Input: part model. Units: mm. Frame: model coordinates. A direction names the side the tool comes from. Coordinates: 2 decimals unless noted, no trailing zeros. Write each loop counter-clockwise with the first axis right and the second up, starting at its lowest first coordinate (ties: lowest second). Pieces come first, ordered by that corner, then holes.
1) Draft query along Y for faces 1 (the flat face through (21, 0, 21)), 2 (the cylindrical face through (16.16, -14.47, 37.88)), 3 (the cylindrical face through (-2.38, -10.74, 41.09)). Return one class per face: pulls with the +Y half, pulls with the -Y half, needs draft (parallel to the pull), parting line crosses it, or undercut.
2) Set-up query: faces 4 (the flat face through (15, -16, 3)), 5 (the flat face through (23, -8.2, 41)), 6 (the cylindrical face through (16.16, 16.53, 37.88)). Return all of +Z, -Z, +X, -X, +Y, -Y with unobstructed straight access to the full face (end or side cutting, diameter ignored); none if empty.
3) Pin query (flat end, axial travel): pin 1 Ø4.5 at (x, y) = (23.5, 3) entering from -Z; pin 2 Ø3 at (x, z) = (22.5, 42) entering from -Y; pin 3 Ø5 at (x, z) = (17, 39.5) entering from +Y; pin 4 Ø6.5 at (x, y) = (24, -2.5) entering from +Z. Return the tip coordinate at first contact, or that it passes through.
4) Section query D-D (x = 0). Output: boundary loops of the cut face in (y, z).
5) Section query A-A (y = -15.5). Output: boundary loops of the cut face in (x, z) (3 decimals).
6) Line query: L1, parallel to Y at x = 15.5, z = 37.2 (3 decimals); L2, parallel to X at y = 15.5, z = 2.2; L3, parallel to X at y = 15, z = 2. Output: solid intervals per line, ascending.
7) Section query C-C (y = 12). Output: boundary loops of the cut face in (x, z), then the cut area to 3 significant figures.
from build123d import *

# Parameters (mm, degrees)
BOX_W           = 4
BOX_H           = 0.5
BOX_DEPTH       = 0.5
ARRAY_Y_COUNT   = 6
ARRAY_Y_PITCH   = 2
SKETCH017_W     = 15
SKETCH017_H     = 6.1
PAD008_DEPTH    = 6.7
POCKET007_DEPTH = 4.6
PAD002_DEPTH    = 9.6
PAD003_DEPTH    = 22.75
PAD004_DEPTH    = 7.75
SKETCH010_R     = 1.225
POCKET003_DEPTH = 4.5
SKETCH011_R     = 11
SKETCH011_R_2   = 5
PAD005_DEPTH    = 2
SKETCH012_R     = 2.5
PAD006_DEPTH    = 20
SKETCH013_W     = 0.5
SKETCH013_H     = 3
POCKET004_DEPTH = 17
SKETCH014_R     = 1.5
SKETCH014_R_2   = 4.5
POCKET005_DEPTH = 3
CHAMFER004_SIZE = 0.4
SKETCH015_W     = 4.3
SKETCH015_H     = 16.4
PAD007_DEPTH    = 3.6
SKETCH016_W     = 16.4
SKETCH016_H     = 6
POCKET006_DEPTH = 1


with BuildPart() as pins:
    # Box → Box (new body)
    with BuildSketch(Plane.XY):
        with Locations((2, 0.25)):
            Rectangle(BOX_W, BOX_H)
    extrude(amount=BOX_DEPTH)

    # Array Y: pins ×6


with BuildPart() as pins_1:
    add(pins.part)
    with Locations(*[(0, i * ARRAY_Y_PITCH, 0) for i in range(1, ARRAY_Y_COUNT)]):
        add(pins.part)


with BuildPart() as pins_2:
    # Array placement: moved
    add(pins_1.part.moved(Location((2, -5.3, 0))))


with BuildPart() as connector:
    # Sketch017 → Pad008 (new body)
    with BuildSketch(Plane.YZ):
        Rectangle(SKETCH017_W, SKETCH017_H)
    extrude(amount=PAD008_DEPTH)

    # Sketch018 (on Face6 of Pad008) → Pocket007 (cut)
    with BuildSketch(Plane.YZ.offset(6.7)):
        Polygon((-6.5, 1.85), (-3.227377, 1.85), (-3.227377, 3.85), (3.227377, 3.85), (3.227377, 1.85), (6.5, 1.85), (6.5, -1.85), (-6.5, -1.85), align=None)
    extrude(amount=-POCKET007_DEPTH, mode=Mode.SUBTRACT)

    # Fusion001: union pins
    add(pins_2.part)


with BuildPart() as connector_1:
    # Fusion001 placement: moved
    add(connector.part.moved(Location((20.15, 0, 6.65))))


with BuildPart() as motor_with_connector:
    # Sketch007 → Pad002 (new body)
    with BuildSketch(Plane.XY):
        with BuildLine():
            Line((-16.65, -21.15), (16.65, -21.15))
            ThreePointArc((16.65, -21.15), (19.033457, -19.033457), (21.15, -16.65))
            Line((21.15, -16.65), (21.15, 16.65))
            ThreePointArc((21.15, 16.65), (19.033457, 19.033457), (16.65, 21.15))
            Line((16.65, 21.15), (-16.65, 21.15))
            ThreePointArc((-16.65, 21.15), (-19.033457, 19.033457), (-21.15, 16.65))
            Line((-21.15, 16.65), (-21.15, -16.65))
            ThreePointArc((-21.15, -16.65), (-19.033457, -19.033457), (-16.65, -21.15))
        make_face()
    extrude(amount=PAD002_DEPTH)

    # Sketch008 (on Face10 of Pad002) → Pad003 (new body)
    with BuildSketch(Plane.XY.offset(9.6)):
        Polygon((-21, -13.75), (-21, 13.75), (-13.75, 21), (13.75, 21), (21, 13.75), (21, -13.75), (13.75, -21), (-13.75, -21), align=None)
    extrude(amount=PAD003_DEPTH)

    # Sketch009 (on Face19 of Pad003) → Pad004 (new body)
    with BuildSketch(Plane.XY.offset(32.35)):
        with BuildLine():
            Line((-16.65, -21.15), (16.65, -21.15))
            ThreePointArc((16.65, -21.15), (19.033457, -19.033457), (21.15, -16.65))
            Line((21.15, -16.65), (21.15, 16.65))
            ThreePointArc((21.15, 16.65), (19.033457, 19.033457), (16.65, 21.15))
            Line((16.65, 21.15), (-16.65, 21.15))
            ThreePointArc((-16.65, 21.15), (-19.033457, 19.033457), (-21.15, 16.65))
            Line((-21.15, 16.65), (-21.15, -16.65))
            ThreePointArc((-21.15, -16.65), (-19.033457, -19.033457), (-16.65, -21.15))
        make_face()
    extrude(amount=PAD004_DEPTH)

    # Sketch010 (on Face28 of Pad004) → Pocket003 (cut)
    with BuildSketch(Plane.XY.offset(40.1)):
        with Locations((-15.5, 15.5)):
            Circle(SKETCH010_R)
        with Locations((15.5, 15.5)):
            Circle(SKETCH010_R)
        with Locations((15.5, -15.5)):
            Circle(SKETCH010_R)
        with Locations((-15.5, -15.5)):
            Circle(SKETCH010_R)
    extrude(amount=-POCKET003_DEPTH, mode=Mode.SUBTRACT)

    # Sketch011 (on Face28 of Pocket003) → Pad005 (new body)
    with BuildSketch(Plane.XY.offset(40.1)):
        Circle(SKETCH011_R)
        Circle(SKETCH011_R_2, mode=Mode.SUBTRACT)
    extrude(amount=PAD005_DEPTH)

    # Sketch012 (on Face40 of Pad005) → Pad006 (new body)
    with BuildSketch(Plane.XY.offset(40.1)):
        Circle(SKETCH012_R)
    extrude(amount=PAD006_DEPTH)

    # Sketch013 (on Face42 of Pad006) → Pocket004 (cut)
    with BuildSketch(Plane.XY.offset(60.1)):
        with Locations((-2.25, 0)):
            Rectangle(SKETCH013_W, SKETCH013_H)
    extrude(amount=-POCKET004_DEPTH, mode=Mode.SUBTRACT)

    # Sketch014 (on Face4 of Pocket004) → Pocket005 (cut)
    with BuildSketch(Plane(origin=(0, 0, 0), x_dir=(1, 0, 0), z_dir=(0, 0, -1))):
        with Locations((-15.5, 15.5)):
            Circle(SKETCH014_R)
        with Locations((15.5, 15.5)):
            Circle(SKETCH014_R)
        with Locations((15.5, -15.5)):
            Circle(SKETCH014_R)
        with Locations((-15.5, -15.5)):
            Circle(SKETCH014_R)
        Circle(SKETCH014_R_2)
    extrude(amount=-POCKET005_DEPTH, mode=Mode.SUBTRACT)

    # Chamfer004
    chamfer004_edges = [motor_with_connector.edges().sort_by_distance(p)[0] for p in [
        (-16.725, 15.5, 35.6),
    ]]
    chamfer(chamfer004_edges, length=CHAMFER004_SIZE)

    # Sketch015 (on Face45 of Chamfer004) → Pad007 (new body)
    with BuildSketch(Plane.XY.offset(43.1)):
        with Locations((23.3, 0)):
            Rectangle(SKETCH015_W, SKETCH015_H)
    extrude(amount=-PAD007_DEPTH)

    # Sketch016 (on Face5 of Pad007) → Pocket006 (cut)
    with BuildSketch(Plane(origin=(21.15, 0, 0), x_dir=(0, -1, 0), z_dir=(-1, 0, 0))):
        with Locations((0, 6.6)):
            Rectangle(SKETCH016_W, SKETCH016_H)
    extrude(amount=-POCKET006_DEPTH, mode=Mode.SUBTRACT)

    # Fusion002: union connector
    add(connector_1.part)


solid = motor_with_connector.part
Answer:
1. face 1: needs draft
1. face 2: undercut
1. face 3: parting line crosses it
2. face 4: -Z
2. face 5: +Z, -Z, +X, -Y
2. face 6: +Z
3. pin 1: stops at z = 3.6
3. pin 2: stops at y = -8.2
3. pin 3: stops at y = 21.15
3. pin 4: stops at z = 43.1
4. outline: (-21.15, 0) - (-4.5, 0) - (-4.5, 3) - (4.5, 3) - (4.5, 0) - (21.15, 0) - (21.15, 9.6) - (21, 9.6) - (21, 32.35) - (21.15, 32.35) - (21.15, 40.1) - (11, 40.1) - (11, 42.1) - (5, 42.1) - (5, 40.1) - (2.5, 40.1) - (2.5, 60.1) - (-2.5, 60.1) - (-2.5, 40.1) - (-5, 40.1) - (-5, 42.1) - (-11, 42.1) - (-11, 40.1) - (-21.15, 40.1) - (-21.15, 32.35) - (-21, 32.35) - (-21, 9.6) - (-21.15, 9.6) - close
5. outline: (-21.15, 0) - (-17, 0) - (-17, 3) - (-14, 3) - (-14, 0) - (14, 0) - (14, 3) - (17, 3) - (17, 0) - (21.15, 0) - (21.15, 9.6) - (19.25, 9.6) - (19.25, 32.35) - (21.15, 32.35) - (21.15, 40.1) - (16.725, 40.1) - (16.725, 35.6) - (14.275, 35.6) - (14.275, 40.1) - (-14.275, 40.1) - (-14.275, 35.6) - (-16.725, 35.6) - (-16.725, 40.1) - (-21.15, 40.1) - (-21.15, 32.35) - (-19.25, 32.35) - (-19.25, 9.6) - (-21.15, 9.6) - close
6. L1: y = -21.15 to -16.725, -14.275 to 14.275, 16.725 to 21.15
6. L2: x = -21.15 to -17, -14 to 14, 17 to 21.15
6. L3: x = -21.15 to -16.91, -14.09 to 14.09, 16.91 to 21.15
7. outline: (-21.15, 0) - (21.15, 0) - (21.15, 9.6) - (21, 9.6) - (21, 32.35) - (21.15, 32.35) - (21.15, 40.1) - (-21.15, 40.1) - (-21.15, 32.35) - (-21, 32.35) - (-21, 9.6) - (-21.15, 9.6) - close
7. area: 1,690 mm2
